from build123d import *

# Parameters (mm, degrees)
F1_DEPTH = 9
F0_R     = 5.5
F2_DEPTH = 5
F3_W     = 2.5
F3_H     = 8
F5_R     = 1
F6_DEPTH = 12.5


with BuildPart() as f1:
    # F0 (on Top) → F1 (new body)
    with BuildSketch(Plane.XY):
        Polygon((0, 2.8867513459), (-2.5, 1.443375673), (-2.5, -1.443375673), (0, -2.8867513459), (2.5, -1.443375673), (2.5, 1.443375673), align=None)
    extrude(amount=F1_DEPTH)

    # F0 (on Top) → F2 (join)
    with BuildSketch(Plane.XY):
        Circle(F0_R)
        Polygon((-2.5, -1.443375673), (-2.5, 1.443375673), (0, 2.8867513459), (2.5, 1.443375673), (2.5, -1.443375673), (0, -2.8867513459), align=None, mode=Mode.SUBTRACT)
    extrude(amount=F2_DEPTH)

    # F3 (on Right) → F4 (revolve, cut)
    with BuildSketch(Plane.YZ):
        with Locations((1.25, 0)):
            Rectangle(F3_W, F3_H)
    revolve(axis=Axis((0, 0, -0.2936716191), (0, 0, -1)), mode=Mode.SUBTRACT)

    # F5 (on Right) → F6 (cut, symmetric)
    with BuildSketch(Plane.YZ):
        with Locations((0, 2)):
            Circle(F5_R)
    extrude(amount=F6_DEPTH, both=True, mode=Mode.SUBTRACT)


solid = f1.part
For this review, take the finished solid that the model builds, in its own axes (mm). A direction names the side the tool comes from. Round coordinates to 2 decimals unless told otherwise and drop trailing zeros. Write each loop counter-clockwise with the first axis right and the second up, starting at its lowest first coordinate (ties: lowest second). Pieces come first, ordered by that corner, then holes. Notation, with made-up numbers: (19.5, 89) -> (49.5, 89) arc R15 cw to (49.5, 118) -> close; hole circle Ø5 at (76, -25.75). An arc over 180 degrees is marked (long way). Put each result on its own line as item: value.
Q1. Consider section D-D on x = 0.25. State the section outline as (y, z) points, and give its area (3 significant figures).
Determined:
outline: (-5.49, 0) -> (-2.49, 0) -> (-2.49, 4) -> (2.49, 4) -> (2.49, 0) -> (5.49, 0) -> (5.49, 5) -> (2.74, 5) -> (2.74, 9) -> (-2.74, 9) -> (-2.74, 5) -> (-5.49, 5) -> close
area: 57.0 mm^2
Q2. Clearance check with flat-ended pins moving along their axes: pin 1 Ø5 at (x, y) = (4.5, -4) entering from +Z; pin 2 Ø5.5 at (x, y) = (-1, -1) entering from -Z; pin 3 Ø0.9 at (y, z) = (0, 6.5) entering from -X; pin 4 Ø1 at (x, z) = (4, 4) entering from -Y. State where each tip first meets the part, or that it passes through.
Determined:
pin 1: stops at z = 5
pin 2: stops at z = 0
pin 3: stops at x = -2.5
pin 4: stops at y = -4.24
Q3. Consider section B-B on z = 2.75. State the section outline as (x, y) points, and give its area (3 significant figures).
Determined:
outline: (-5.46, -0.66) arc R5.5 ccw to (5.46, -0.66) -> (2.41, -0.66) arc R2.5 cw to (-2.41, -0.66) -> close; (-5.46, 0.66) -> (-2.41, 0.66) arc R2.5 cw to (2.41, 0.66) -> (5.46, 0.66) arc R5.5 ccw to start
area: 67.4 mm^2
Q4. To check wall thickness, follow L1, parallel to Y at x = 0, z = 2.05; L2, parallel to Z at x = -4.6, y = 0; L3, parallel to X at y = 5, z = 4.25. State the ranges of each line that lie inside material, in increasing order. Write a range as [from, to].
Determined:
L1: y = [-5.5, -2.5], [2.5, 5.5]
L2: z = [0, 1], [3, 5]
L3: x = [-2.29, 2.29]
Q5. Consider section C-C on z = 3.75. State the section outline as (x, y) points.
Determined:
outline: circle Ø11 at (0, 0); hole circle Ø5 at (0, 0)
Q6. Consider section A-A on y = 0. State the section outline as (x, z) points.
Determined:
outline: (-5.5, 0) -> (-2.5, 0) -> (-2.5, 1) -> (-5.5, 1) -> close; (-5.5, 3) -> (-2.5, 3) -> (-2.5, 4) -> (2.5, 4) -> (2.5, 3) -> (5.5, 3) -> (5.5, 5) -> (2.5, 5) -> (2.5, 9) -> (-2.5, 9) -> (-2.5, 5) -> (-5.5, 5) -> close; (2.5, 0) -> (5.5, 0) -> (5.5, 1) -> (2.5, 1) -> close
Q7. Machinability: for faces 4 (the flat face through (-3, 0, 5)), 5 (the flat face through (-2.5, 0, 7)), 6 (the flat face through (-1.233, 2.175, 6.972)), which of the approach directions +Z, -Z, +X, -X, +Y, -Y give a long, thin tool a straight path to every point of the face, cutting with its end or side? Answer none if there is none.
Determined:
face 4: +Z
face 5: +Z, -X, +Y, -Y
face 6: +Z, -X, +Y
Q8. The part is to be moulded in two halves that separate along X. For faces 1 (the flat face through (1.267, 2.155, 6.972)), 2 (the cylindrical face through (-2.22, 1.15, 2.03)), 3 (the cylindrical face through (5.08, -2.11, 2.46)), say which applies: released by +X, released by -X, zero draft, split by the parting line, or undercut.
Determined:
face 1: released by +X
face 2: undercut
face 3: split by the parting line
